Model file for the job. Use its own axes, mm. Coordinates: 2 decimals unless noted, no trailing zeros. Write each loop counter-clockwise with the first axis right and the second up, starting at its lowest first coordinate (ties: lowest second). Pieces come first, ordered by that corner, then holes. Notation, with made-up numbers: M 69,3.5 L 84,3.5 A15 cw 84,29.5 Z; hole C 33.5,38 d9. An arc over 180 degrees is marked long. One line per question, with ' | ' between items. Start each with the question number.
(1) Cut at A-A (y = 51.5). Write the cut outline in (x, z) (3 decimals).
(2) Flat gauge pin, fed straight in: pin 1 Ø2 at (x, y) = (193, 69) entering from +Z (3 decimals). Where does the tip first touch, or does it go through?
(3) Wall check: probe 1 along Z at (x, y) = (191.5, 57) (3 decimals); probe 2 along Z at (x, y) = (192, 74) (3 decimals); probe 3 along Z at (x, y) = (195, 52.5). Give the ranges that are in metal, low to high.
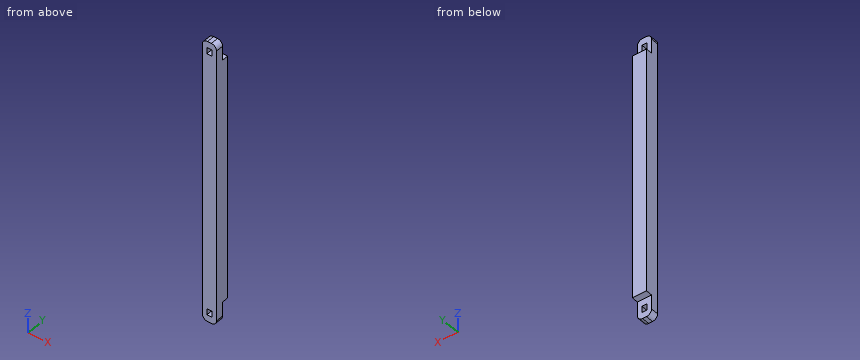
from build123d import *

# Parameters (mm, degrees)
SKETCH1_W           = 34.925
SKETCH1_H           = 34.925
BOSS_EXTRUDE1_DEPTH = 698.5
SKETCH2_W           = 47.625
SKETCH2_H           = 15.875
CUT_EXTRUDE1_DEPTH  = 127
SKETCH3_W           = 12.7
SKETCH3_H           = 15.24
CUT_EXTRUDE2_DEPTH  = 728.836573147
FILLET1_R           = 12.7


with BuildPart() as part:
    # Sketch1 → Boss-Extrude1 (new body)
    with BuildSketch(Plane.XY):
        with Locations((186.206164037, 61.261572703)):
            Rectangle(SKETCH1_W, SKETCH1_H)
    extrude(amount=BOSS_EXTRUDE1_DEPTH)

    # Sketch2 → Cut-Extrude1 (cut)
    with BuildSketch(Plane(origin=(203.668664037, 0, 0), x_dir=(0, 0, -1), z_dir=(1, 0, 0))):
        with Locations((-23.8125, 70.786572703)):
            Rectangle(SKETCH2_W, SKETCH2_H)
        with Locations((-674.6875, 70.786572703)):
            Rectangle(SKETCH2_W, SKETCH2_H)
    extrude(amount=-CUT_EXTRUDE1_DEPTH, mode=Mode.SUBTRACT)

    # Sketch3 → Cut-Extrude2 (cut, through all)
    with BuildSketch(Plane(origin=(0, 62.849072703, 0), x_dir=(1, 0, 0), z_dir=(0, 1, 0))):
        with Locations((186.206164037, -675.005)):
            Rectangle(SKETCH3_W, SKETCH3_H)
        with Locations((186.206164037, -23.495)):
            Rectangle(SKETCH3_W, SKETCH3_H)
    extrude(amount=-CUT_EXTRUDE2_DEPTH, mode=Mode.SUBTRACT)

    # Fillet1
    fillet1_edges = [part.edges().sort_by_distance(p)[0] for p in [
        (203.668664037, 53.324072703, 698.5),
        (168.743664037, 53.324072703, 698.5),
        (168.743664037, 53.324072703, 0),
        (203.668664037, 53.324072703, 0),
    ]]
    fillet(fillet1_edges, radius=FILLET1_R)


solid = part.part
Filled in:
1) outline: M 168.744,12.7 A12.7 ccw 181.444,0 L 190.969,0 A12.7 ccw 203.669,12.7 L 203.669,685.8 A12.7 ccw 190.969,698.5 L 181.444,698.5 A12.7 ccw 168.744,685.8 Z; hole M 179.856,15.875 L 192.556,15.875 L 192.556,31.115 L 179.856,31.115 Z; hole M 179.856,667.385 L 192.556,667.385 L 192.556,682.625 L 179.856,682.625 Z
2) pin 1: z = 650.875
3) probe 1: 0.011 to 15.875, 31.115 to 667.385, 682.625 to 698.489 | probe 2: 47.625 to 650.875 | probe 3: 0.66 to 697.84
